Study the drawing (mm; zero at the part's minimum x, y, z) and answer. Coordinates: 2 decimals unless noted, no trailing zeros. Loops run counter-clockwise (first coordinate to the right, second up) from the corner with the lowest first, then second, coordinate; pieces in that order, holes last. Notation, with made-up numbers: (6.5, -3) -> (50.5, -3) arc R10 cw to (50.5, 2) -> close; hole circle Ø3 at (88.5, -36). An arc over 180 degrees is marked (long way). Answer as a JSON object with one key per item and string values. Group by question number.
Q1. This flat-tipped pin is pushed along its axis until it touches: P1, Ø6, axis at x = 7.5, y = 30, coming from the -Z side. Where does it stop, or does it pass through?
Q2. The part is cut by section B-B on x = 42.5. Write down the section's boundary in (y, z).
Q3. The part is cut by section C-C on z = 1.85. Write down the section's boundary in (x, y), and give its area (3 significant figures).
Q4. Straight lines are drawn through the part: line 1 along Y through (x, z) = (7.5, 2.3); line 2 along X through (y, z) = (8, 5.25); line 3 along X through (y, z) = (7, 1.45). For each, find the intervals that lie inside material, in ascending order. Write a range as [from, to].
Q5. The part is cut by section A-A on y = 30. Write down the section's boundary in (x, z), and give its area (4 significant figures).
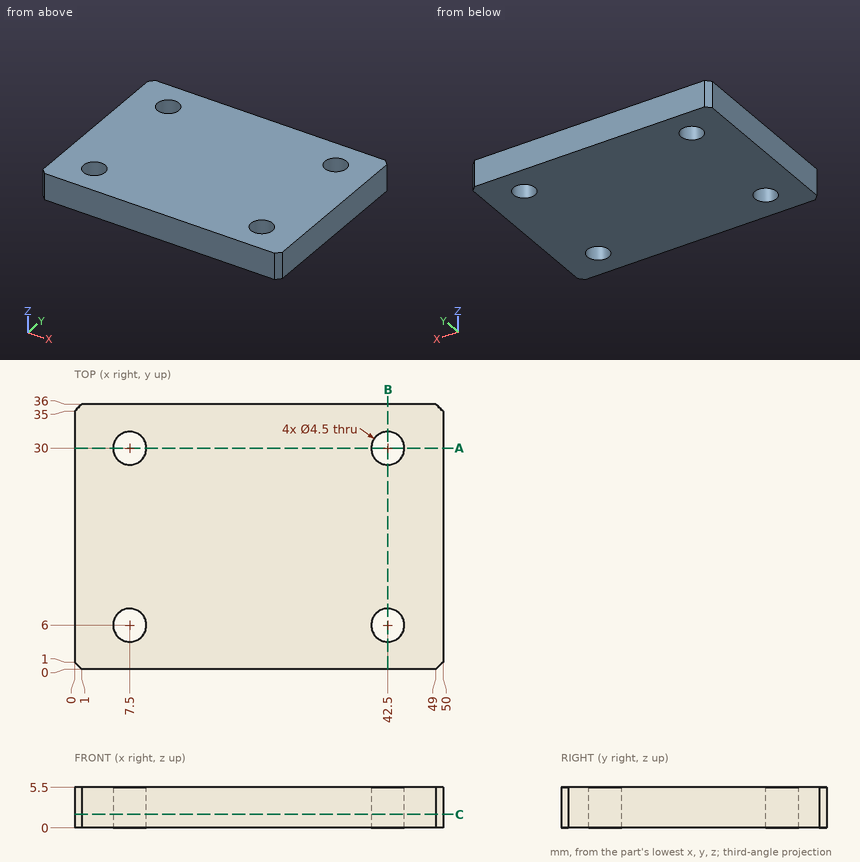
Final values:
{
 "1": {"P1": "stops at z = 0"},
 "2": {"outline": "(0, 0) -> (3.75, 0) -> (3.75, 5.5) -> (0, 5.5) -> close; (8.25, 0) -> (27.75, 0) -> (27.75, 5.5) -> (8.25, 5.5) -> close; (32.25, 0) -> (36, 0) -> (36, 5.5) -> (32.25, 5.5) -> close"},
 "3": {"outline": "(0, 1) -> (1, 0) -> (49, 0) -> (50, 1) -> (50, 35) -> (49, 36) -> (1, 36) -> (0, 35) -> close; hole circle Ø4.5 at (7.5, 6); hole circle Ø4.5 at (7.5, 30); hole circle Ø4.5 at (42.5, 6); hole circle Ø4.5 at (42.5, 30)", "area": "1,730 mm2"},
 "4": {"line 1": "y = [0, 3.75], [8.25, 27.75], [32.25, 36]", "line 2": "x = [0, 6.47], [8.53, 41.47], [43.53, 50]", "line 3": "x = [0, 5.48], [9.52, 40.48], [44.52, 50]"},
 "5": {"outline": "(0, 0) -> (5.25, 0) -> (5.25, 5.5) -> (0, 5.5) -> close; (9.75, 0) -> (40.25, 0) -> (40.25, 5.5) -> (9.75, 5.5) -> close; (44.75, 0) -> (50, 0) -> (50, 5.5) -> (44.75, 5.5) -> close", "area": "225.5 mm2"}
}
